Here's how the part is built. I have some questions about the finished solid (model axes, mm). Round coordinates to 2 decimals unless told otherwise and drop trailing zeros. Loops run counter-clockwise (first coordinate to the right, second up) from the corner with the lowest first, then second, coordinate; pieces in that order, holes last. Notation, with made-up numbers: (47, -24.5) - (83, -24.5) arc R20 ccw to (83, -9.5) - close; hole circle Ø7 at (64.25, -1.75). An arc over 180 degrees is marked (long way). Return JSON: item names as keys, results as strings. Group by question number.
```python
from build123d import *

# Parameters (mm, degrees)
SKETCH_1_W          = 20
SKETCH_1_H          = 20
EXTRUDE_1_DEPTH     = 58
SKETCH_2_R          = 2.75
CUT_EXTRUDE_1_DEPTH = 63.161081072


with BuildPart() as part:
    # 草图1 → 凸台-拉伸1 (new body)
    with BuildSketch(Plane.XY):
        Rectangle(SKETCH_1_W, SKETCH_1_H)
    extrude(amount=EXTRUDE_1_DEPTH)

    # 草图2 → 切除-拉伸1 (cut, through all)
    with BuildSketch(Plane(origin=(0, 10, 0), x_dir=(1, 0, 0), z_dir=(0, 1, 0))):
        with Locations(Location((0, -6, 0), (0, 0, 270))):
            Circle(SKETCH_2_R)
        with Locations(Location((0, -52, 0), (0, 0, 90))):
            Circle(SKETCH_2_R)
    extrude(amount=-CUT_EXTRUDE_1_DEPTH, mode=Mode.SUBTRACT)


solid = part.part
```
Q1. Imagine slicing it at D-D, the plane z = 6.5. List the corners of the cut face in (x, y) for me.
Q2. If we mould it in two halves opening along X, with no side actions, what happens to faces 1 (the flat face through (10, 0, 29)), 2 (the flat face through (0, 0, 0)), 3 (the cylindrical face through (-0.121, 0.14, 54.747))? For each: +X half, -X half, draft (parallel to the pull), parting line (faces both ways), or undercut.
Q3. Imagine slicing it at C-C, the plane x = 0. List the corners of the cut face in (y, z) for me, and give its area (3 significant figures).
Q4. Please list where these lines run through material, in increasing order: line 1 (X direction, y = 3.5, z = 6); line 2 (Z direction, x = -0.5, y = -3).
Q5. Imagine slicing it at B-B, the plane y = 3.75. List the corners of the cut face in (x, z) for me.
Q6. Imagine slicing it at A-A, the plane z = 52. List the corners of the cut face in (x, y) for me, and give its area (3 significant figures).
Output values:
{
 "1": {"outline": "(-10, -10) - (-2.7, -10) - (-2.7, 10) - (-10, 10) - close; (2.7, -10) - (10, -10) - (10, 10) - (2.7, 10) - close"},
 "2": {"face 1": "+X half", "face 2": "draft", "face 3": "undercut"},
 "3": {"outline": "(-10, 0) - (10, 0) - (10, 3.25) - (-10, 3.25) - close; (-10, 8.75) - (10, 8.75) - (10, 49.25) - (-10, 49.25) - close; (-10, 54.75) - (10, 54.75) - (10, 58) - (-10, 58) - close", "area": "940 mm^2"},
 "4": {"line 1": "x = -10 to -2.75, 2.75 to 10", "line 2": "z = 0 to 3.3, 8.7 to 49.3, 54.7 to 58"},
 "5": {"outline": "(-10, 0) - (10, 0) - (10, 58) - (-10, 58) - close; hole circle Ø5.5 at (0, 6); hole circle Ø5.5 at (0, 52)"},
 "6": {"outline": "(-10, -10) - (-2.75, -10) - (-2.75, 10) - (-10, 10) - close; (2.75, -10) - (10, -10) - (10, 10) - (2.75, 10) - close", "area": "290 mm^2"}
}
